CAD build for the part. Positions are in the model's coordinates, mm. Face numbers are marked on the shaded views. A direction names the side the tool comes from. Round coordinates to 2 decimals unless told otherwise and drop trailing zeros. Write each loop counter-clockwise with the first axis right and the second up, starting at its lowest first coordinate (ties: lowest second). Pieces come first, ordered by that corner, then holes. Notation, with made-up numbers: (39.25, 32) -> (90.25, 32) arc R21 ccw to (90.25, 69) -> close; hole circle Ø5 at (-13, 78.25). An arc over 180 degrees is marked (long way). Put each result on its own line as item: value. Start each with the question number.
1. Saw through at A-A on x = 32. List the corners of the cut face in (y, z), and give its area (3 significant figures).
2. Saw through at B-B on z = 32. List the corners of the cut face in (x, y), and give its area (3 significant figures).
3. Saw through at D-D on z = 23. List the corners of the cut face in (x, y), and give its area (3 significant figures).
4. Saw through at C-C on y = 10. List the corners of the cut face in (x, z).
5. Drill centre lines: line 1 (Y direction, x = 10.5, z = 21); line 2 (Z direction, x = 2.8, y = 10); line 3 (Y direction, x = 19, z = 1). Where is each one in solid material? Low to high. Write a range as from..to.
6. Flat gauge pins, fed straight in: P1, Ø2, axis at x = 15, y = 12.5, coming from the +Z side; P2, Ø5, axis at y = 12, z = 14.5, coming from the +X side; P3, Ø2, axis at x = 7, y = 10, coming from the -Z side. Where does each tip first touch, or does it go through?
7. 3-axis set-ups, long thin cutter, end or side, ignore diameter. For the marked faces 4 and 5: which of +Z, -Z, +X, -X, +Y, -Y reach the whole face in a straight line?
8. Pull direction Y, two halves, no side cores. Call the marked faces 1, 2 and 3: pulls with the +Y half, pulls with the -Y half, needs draft (parallel to the pull), parting line crosses it, or undercut.
Autodesk Fusion 360 part; units mm, degrees
sketch "Sketch5" plane through (0, 0, 0) normal (0, 1, 0) x (1, 0, 0)
  line L0 (0, -9) -> (0, -42)
  line L1 (5, -41) -> (5, -37)
  line L2 (4, -42) -> (0, -42)
  line L3 (5, -37) -> (37, -5)
  line L4 (37, -5) -> (41, -5)
  line L5 (42, -4) -> (42, 0)
  arc A0 (4, -42) -> (5, -41) centre (4, -41) ccw
  arc A1 (41, -5) -> (42, -4) centre (41, -4) ccw
  line L6 (0, -9) -> (9, 0)
  line L7 (42, 0) -> (9, 0)
  line L8 (5, -37) -> (5, -11.0711)
  line L9 (5, -11.0711) -> (11.0711, -5)
  line L10 (11.0711, -5) -> (37, -5)
  point P0 (5, -42)
  point P1 (42, -5)
  dimension "d59" = 5
  dimension "d60" = 5
  dimension "d61" = 1
  dimension "d65" = 5
  dimension "d89" = 135
  dimension "d90" = 42
  dimension "d91" = 42
  dimension "d92" = 5
  dimension "d93" = 9
extrude "Extrude14" add sketch "Sketch5" along normal blind 4
extrude "Extrude15" add sketch "Sketch5" along normal blind 20 contours L0 L1 L2 L4 L5 A0 A1 L6 L7 L8 L9 L10
extrude "Extrude16" add sketch "Sketch5" against normal blind 4 from surface at 20
sketch "Sketch6" plane through (0, 0, 5) normal (0, 0, 1) x (-1, 0, 0)
  line L0 (-37, -16) -> (-11.0711, -16)
  line L1 (-11.0711, -16) -> (-11.0711, -4)
  line L2 (-11.0711, -4) -> (-37, -4)
  circle A0 centre (-19, -10) radius 2.5
  circle A1 centre (-32, -10) radius 2.5
  line L3 (-42, 0) -> (-42, -20)
  line L4 (-37, -20) -> (-5, -20)
  line L5 (-37, -4) -> (-37, 0)
  line L6 (-37, 0) -> (-41, 0)
  line L7 (-41, 0) -> (-41, -20)
  line L8 (-41, -20) -> (-37, -20)
  line L9 (-37, -20) -> (-37, -16)
  dimension "d71" = 5
  dimension "d72" = 10
  dimension "d73" = 13
  dimension "d74" = 10
sketch "Sketch7" plane through (5, 0, 0) normal (1, 0, 0) x (0, 1, 0)
  line L0 (20, 41) -> (0, 41)
  line L1 (0, 41) -> (0, 37)
  line L2 (0, 37) -> (4, 37)
  line L3 (4, 37) -> (4, 11.0711)
  line L4 (4, 11.0711) -> (16, 11.0711)
  line L5 (16, 11.0711) -> (16, 37)
  line L6 (16, 37) -> (20, 37)
  line L7 (20, 37) -> (20, 41)
  circle A0 centre (10, 32) radius 2.5
  circle A1 centre (10, 19) radius 2.5
  line L8 (0, 42) -> (20, 42)
  line L9 (0, 37) -> (0, 5)
  dimension "d75" = 5
  dimension "d76" = 10
  dimension "d77" = 13
  dimension "d78" = 10
extrude "Extrude17" cut sketch "Sketch7" against normal through all contours A0 | A1
extrude "Extrude18" cut sketch "Sketch6" against normal through all contours A0 | A1
fillet "Fillet5" radius 1 2 edges at (5, 10, 11.0711) (11.0711, 10, 5)
fillet "Fillet6" radius 1 4 edges at (37, 2, 5) (5, 2, 37) (5, 18, 37) (37, 18, 5)
sketch "Sketch8" plane through (0, 0, 0) normal (0, 0, -1) x (1, 0, 0)
  line L0 (42, -20) -> (42, 0)
  line L1 (42, 0) -> (9, 0)
  line L2 (9, 0) -> (9, -20)
  line L3 (9, -20) -> (42, -20)
  line L4 (42, -10) -> (9, -10) construction
  line L5 (42, -6.925) -> (38, -6.925)
  line L6 (38, -6.925) -> (38, -13.075)
  line L7 (38, -13.075) -> (42, -13.075)
  line L8 (42, -13.075) -> (42, -6.925)
  circle A0 centre (19, -10) radius 2.5
  circle A1 centre (32, -10) radius 2.5
  dimension "d87" = 6.15
  dimension "d88" = 4
sketch "Sketch9" plane through (0, 0, 0) normal (-1, 0, 0) x (0, -1, 0)
  circle A0 centre (-10, 32) radius 2.5
  circle A1 centre (-10, 19) radius 2.5
  line L0 (-20, 9) -> (0, 9)
  line L1 (0, 9) -> (0, 42)
  line L2 (0, 42) -> (-20, 42)
  line L3 (-20, 42) -> (-20, 9)
  line L4 (-13.075, 42) -> (-6.925, 42)
  line L5 (-6.925, 42) -> (-6.925, 38)
  line L6 (-6.925, 38) -> (-13.075, 38)
  line L7 (-13.075, 38) -> (-13.075, 42)
  line L8 (-10, 42) -> (-10, 9) construction
  dimension "d98" = 6.15
  dimension "d99" = 4
sketch "Sketch10" plane through (5, 0, 0) normal (1, 0, 0) x (0, 1, 0)
  line L0 (16, 37.4142) -> (20, 37.4142)
  line L1 (20, 37.4142) -> (20, 41)
  line L2 (20, 41) -> (0, 41)
  line L3 (0, 41) -> (0, 37.4142)
  line L4 (0, 37.4142) -> (4, 37.4142)
  line L5 (4, 37.4142) -> (4, 11.4853)
  line L6 (4, 11.4853) -> (16, 11.4853)
  line L7 (16, 11.4853) -> (16, 37.4142)
  circle A0 centre (10, 32) radius 2.5
  circle A1 centre (10, 19) radius 2.5
  circle A2 centre (10, 32) radius 2.6
  circle A3 centre (10, 19) radius 2.6
  dimension "d104" = 5.2
  dimension "d105" = 5.2
extrude "Extrude21" cut sketch "Sketch10" against normal through all contours A0 | A1 | A2 | A3
sketch "Sketch11" plane through (0, 0, 5) normal (0, 0, 1) x (-1, 0, 0)
  circle A0 centre (-32, -10) radius 2.5
  circle A1 centre (-19, -10) radius 2.5
  line L0 (-37.4142, -20) -> (-37.4142, -16)
  line L1 (-37.4142, -16) -> (-11.4853, -16)
  line L2 (-11.4853, -16) -> (-11.4853, -4)
  line L3 (-11.4853, -4) -> (-37.4142, -4)
  line L4 (-37.4142, -4) -> (-37.4142, 0)
  line L5 (-37.4142, 0) -> (-41, 0)
  line L6 (-41, 0) -> (-41, -20)
  line L7 (-41, -20) -> (-37.4142, -20)
  circle A2 centre (-19, -10) radius 2.6
  circle A3 centre (-32, -10) radius 2.6
  dimension "d107" = 5.2
  dimension "d108" = 5.2
extrude "Extrude22" cut sketch "Sketch11" against normal through all contours A0 | A1 | A2 | A3
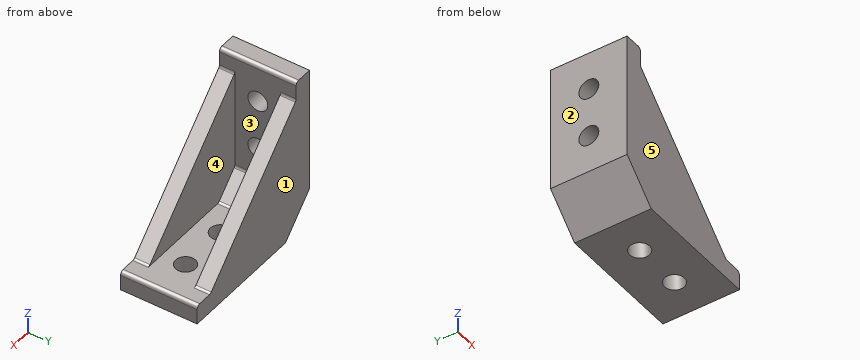
Return value:
1. outline: (0, 0) -> (7.4, 0) -> (7.4, 5) -> (4, 5) -> (4, 10) -> (0, 10) -> close; (12.6, 0) -> (20, 0) -> (20, 10) -> (16, 10) -> (16, 5) -> (12.6, 5) -> close
1. area: 114 mm^2
2. outline: (0, 0) -> (10, 0) -> (10, 4) -> (5, 4) -> (5, 7.4) -> (0, 7.4) -> close; (0, 12.6) -> (5, 12.6) -> (5, 16) -> (10, 16) -> (10, 20) -> (0, 20) -> close
2. area: 114 mm^2
3. outline: (0, 0) -> (19, 0) -> (19, 4) -> (5, 4) -> (5, 16) -> (19, 16) -> (19, 20) -> (0, 20) -> close
3. area: 212 mm^2
4. outline: (0, 9) -> (9, 0) -> (16.4, 0) -> (16.4, 5) -> (11.49, 5) arc R1 cw to (10.78, 5.29) -> (5.29, 10.78) arc R1 cw to (5, 11.49) -> (5, 16.4) -> (0, 16.4) -> close; (0, 21.6) -> (5, 21.6) -> (5, 29.4) -> (0, 29.4) -> close; (0, 34.6) -> (5, 34.6) -> (5, 41) arc R1 ccw to (4, 42) -> (0, 42) -> close; (21.6, 0) -> (29.4, 0) -> (29.4, 5) -> (21.6, 5) -> close; (34.6, 0) -> (42, 0) -> (42, 4) arc R1 ccw to (41, 5) -> (34.6, 5) -> close
5. line 1: y = 0..4, 16..20
5. line 2: z = 6.2..16.4, 21.6..29.4, 34.6..42
5. line 3: y = 0..7.4, 12.6..20
6. P1: stops at z = 5
6. P2: stops at x = 5
6. P3: stops at z = 1
7. face 4: +Z, +X
7. face 5: +Z, -Z, +X, -X, -Y
8. face 1: pulls with the +Y half
8. face 2: needs draft
8. face 3: undercut
